Autodesk Inventor part; units mm, degrees
ref_plane "YZ Plane" through (0, 0, 0) normal (1, 0, 0) x (0, 1, 0)
ref_plane "XZ Plane" through (0, 0, 0) normal (0, 1, 0) x (-1, 0, 0)
ref_plane "XY Plane" through (0, 0, 0) normal (0, 0, 1) x (1, 0, 0)
sketch "Sketch1" plane through (0, 0, 0) normal (0, 1, 0) x (-1, 0, 0)
  circle A0 centre (0, 0) radius 2.5
  dimension "d0" = 5
extrude "Extrusion1" add sketch "Sketch1" along normal blind 20
sketch "Sketch2" plane through (0, 20, 0) normal (0, 1, 0) x (1, 0, 0)
  circle A0 centre (0, 0) radius 2.5
  circle A1 centre (0, 0) radius 5.5
  dimension "d3" = 11
extrude "Extrusion2" add sketch "Sketch2" along normal blind 2.25 contours A0 | A1
sketch "Sketch3" plane through (0, 22.25, 0) normal (0, 1, 0) x (1, 0, 0)
  circle A0 centre (0, 0) radius 5.5
  line L0 (0, 2.217) -> (1.92, 1.1085)
  line L1 (1.92, 1.1085) -> (1.92, -1.1085)
  line L2 (1.92, -1.1085) -> (0, -2.217)
  line L3 (0, -2.217) -> (-1.92, -1.1085)
  line L4 (-1.92, -1.1085) -> (-1.92, 1.1085)
  line L5 (-1.92, 1.1085) -> (0, 2.217)
  dimension "d6" = 1.92
chamfer "Chamfer1" distance 1.75 angle 45 1 edges at (-5.5, 22.25, 0)
sketch "Sketch4" plane through (0, 20, 0) normal (0, -1, 0) x (1, 0, 0)
  circle A0 centre (0, 0) radius 5.5
  circle A1 centre (0, 0) radius 2.5
  circle A2 centre (0, 0) radius 3.5
  dimension "d10" = 7
extrude "Extrusion3" add sketch "Sketch4" along normal blind 0.25 contours A0
extrude "Extrusion4" cut sketch "Sketch3" against normal blind 2 contours L0 L1 L2 L3 L4 L5
thread "Thread1"
properties part number "M5x20BlindScrew" material "Stainless Steel"
The model under review builds one solid part; all positions refer to its coordinate system, in mm. A direction names the side the tool comes from. Give positions to 0.01 mm unless a question says otherwise; leave off trailing zeros. Write each loop counter-clockwise with the first axis right and the second up, starting at its lowest first coordinate (ties: lowest second). Pieces come first, ordered by that corner, then holes.
1. Add section B-B, the plane y = 8.5. Write out the cut boundary in (x, z).
2. Tool access review of faces 1 (the cylindrical face through (-1.19, 20.13, 5.37)), 2 (the flat face through (0, 20.25, 0)), 3 (the flat face through (4, 19.75, 0)): name each direction out of +Z, -Z, +X, -X, +Y, -Y from which nothing blocks a thin tool from reaching the whole face with its end or side.
3. Draft analysis for pull direction Z (two halves, no side actions). For faces 4 (the flat face through (2, 20, 2)), 5 (the flat face through (0, 0, 0)), 6 (the conical face through (-0.5, 22.14, 3.83)), state which applies: +Z half, -Z half, draft (parallel to the pull), parting line (faces both ways), or undercut.
4. Add section A-A, the plane z = 0. Write out the cut boundary in (x, y), plus the area to 3 significant figures.
5. For P1, Ø5, axis at y = 12.5, z = -0.5, coming from the +X side; P2, Ø2, axis at y = 17.5, z = 0, coming from the -X side; P3, Ø1, axis at y = 21.5, z = 0.5, coming from the +X side, all flat-tipped, find the tip position at first contact; note any pin that passes through.
6. Wall thickness on L1, parallel to Z at x = 0, y = 19.95; L2, parallel to Y at x = -2, z = 2.25; L3, parallel to Y at x = 0.5, z = -1.25: over which ranges is each line inside the solid? List them lowest first.
Worked answers:
1. outline: circle Ø5 at (0, 0)
2. face 1: +Y, -Y
2. face 2: +Y
2. face 3: -Y
3. face 4: undercut
3. face 5: draft
3. face 6: parting line
4. outline: (-5.5, 19.75) - (-3.5, 19.75) - (-3.5, 20) - (-2.5, 20) - (-2.5, 0) - (2.5, 0) - (2.5, 20) - (3.5, 20) - (3.5, 19.75) - (5.5, 19.75) - (5.5, 20.5) - (3.75, 22.25) - (1.92, 22.25) - (1.92, 20.25) - (-1.92, 20.25) - (-1.92, 22.25) - (-3.75, 22.25) - (-5.5, 20.5) - close
4. area: 115 mm2
5. P1: stops at x = 2.5
5. P2: stops at x = -2.5
5. P3: stops at x = 4.98
6. L1: z = -5.5 to -3.5, -2.5 to 2.5, 3.5 to 5.5
6. L2: y = 20 to 22.25
6. L3: y = 0 to 20.25
